Part model, mm, in its own coordinate system. Face numbers are marked on the shaded views. Give positions to 0.01 mm unless a question says otherwise; leave off trailing zeros. Write each loop counter-clockwise with the first axis right and the second up, starting at its lowest first coordinate (ties: lowest second). Pieces come first, ordered by that corner, then holes. Notation, with made-up numbers: (43, 70.5) - (76, 70.5) arc R35 ccw to (76, 103.5) - close; hole circle Ø7 at (89.5, 27.25). An arc over 180 degrees is marked (long way). Answer in a Markdown table with one row per item. Add a question column.
1. Band-saw the part on C-C on x = 13. Write the cut outline in (y, z), plus the area to 3 significant figures.
2. Band-saw the part on D-D on y = 15. Write the cut outline in (x, z), plus the area to 3 significant figures.
3. Pull direction X, two halves, no side cores. Call the marked faces 1, 2, 3 and 4: released by +X, released by -X, zero draft, split by the parting line, or undercut.
4. Drop flat-ended pins along their axis: pin 1 Ø8 at (x, y) = (4.5, 30.5) entering from +Z; pin 2 Ø6 at (x, y) = (14.5, 41) entering from +Z. Give the stop position or say it passes through.
5. Probe line 1 along X through (y, z) = (23.5, 11); line 2 along Z through (x, y) = (7.5, 15.5); line 3 along Y through (x, z) = (0.9, 36). List the from-to ranges inside material, lowest first.
6. Band-saw the part on A-A on z = 11.5. Write the cut outline in (x, y), plus the area to 3 significant figures.
7. Band-saw the part on B-B on y = 8. Write the cut outline in (x, z), plus the area to 3 significant figures.
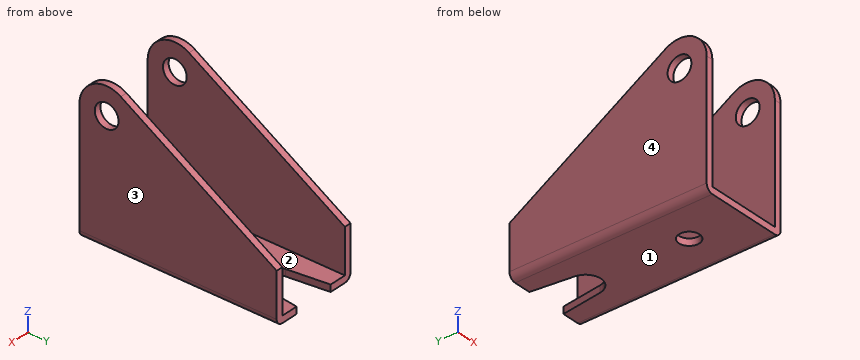
Autodesk Inventor part; units mm, degrees
ref_plane "YZ Plane" through (0, 0, 0) normal (1, 0, 0) x (0, 1, 0)
ref_plane "XZ Plane" through (0, 0, 0) normal (0, 1, 0) x (-1, 0, 0)
ref_plane "XY Plane" through (0, 0, 0) normal (0, 0, 1) x (1, 0, 0)
sketch "Sketch1" plane through (0, 0, 0) normal (0, 0, 1) x (1, 0, 0)
  line L0 (0, 0) -> (26, 0)
  line L1 (26, 0) -> (26, 58)
  line L2 (26, 58) -> (0, 58) construction
  line L3 (0, 58) -> (0, 0)
  circle A0 centre (13, 16) radius 3
  line L4 (0, 58) -> (7, 58)
  line L5 (19, 58) -> (26, 58)
  line L6 (17.464, 45.9318) -> (19, 58)
  line L7 (8.536, 45.9318) -> (7, 58)
  line L8 (13, 58) -> (13, 46.5) construction
  circle A1 centre (13, 46.5) radius 4.5 construction
  arc A2 (8.536, 45.9318) -> (17.464, 45.9318) centre (13, 46.5) ccw
  point P0 (13, 0)
  dimension "d0" = 26
  dimension "d1" = 58
  dimension "d2" = 6
  dimension "d3" = 16
  dimension "d19" = 12
  dimension "d20" = 9
  dimension "d21" = 11.5
extrude "Extrusion1" add sketch "Sketch1" along normal blind 2
sketch "Sketch2" plane through (26, 0, 0) normal (1, 0, 0) x (0, 0, -1)
  circle A0 centre (-36, 8) radius 3.5
  line L0 (0, 0) -> (0, 58)
  line L1 (0, 0) -> (-36, 0)
  circle A1 centre (-36, 8) radius 8 construction
  line L2 (0, 58) -> (-15, 58)
  line L3 (-15, 58) -> (-42.8382, 12.152)
  arc A2 (-42.8382, 12.152) -> (-36, 0) centre (-36, 8) ccw
  dimension "d13" = 16
  dimension "d8" = 7
  dimension "d10" = 8
  dimension "d11" = 36
  dimension "d14" = 15
extrude "Extrusion2" add sketch "Sketch2" against normal blind 2
sketch "Sketch3" plane through (0, 0, 0) normal (-1, 0, 0) x (0, 0, 1)
  line L0 (2, 0) -> (2, 58)
  line L1 (2, 0) -> (36, 0)
  arc A0 (36, 0) -> (42.8382, 12.152) centre (36, 8) ccw
  line L2 (42.8382, 12.152) -> (15, 58)
  line L3 (15, 58) -> (2, 58)
  circle A1 centre (36, 8) radius 3.5
  point P0 (0, 0)
extrude "Extrusion3" add sketch "Sketch3" against normal blind 2
fillet "Fillet1" radius 2 2 edges at (0, 29, 0) (26, 29, 0)
properties part number "Mount" material "Stainless Steel"
Values:
| question | item | result |
|---|---|---|
| 1 | outline | (0, 0) - (13, 0) - (13, 2) - (0, 2) - close; (19, 0) - (42, 0) - (42, 2) - (19, 2) - close |
| 1 | area | 72.0 mm² |
| 2 | outline | (0, 2) arc R2 ccw to (2, 0) - (10.17, 0) - (10.17, 2) - (2, 2) - (2, 41.11) - (0, 41.11) - close; (15.83, 0) - (24, 0) arc R2 ccw to (26, 2) - (26, 41.11) - (24, 41.11) - (24, 2) - (15.83, 2) - close |
| 2 | area | 195 mm² |
| 3 | face 1 | zero draft |
| 3 | face 2 | undercut |
| 3 | face 3 | released by +X |
| 3 | face 4 | released by -X |
| 4 | pin 1 | stops at z = 33.59 |
| 4 | pin 2 | stops at z = 2 |
| 5 | line 1 | x = 0 to 2, 24 to 26 |
| 5 | line 2 | z = 0 to 2 |
| 5 | line 3 | y = 0 to 4.5, 11.5 to 23.41 |
| 6 | outline | (0, 0) - (2, 0) - (2, 58) - (0, 58) - close; (24, 0) - (26, 0) - (26, 58) - (24, 58) - close |
| 6 | area | 232 mm² |
| 7 | outline | (0, 2) arc R2 ccw to (2, 0) - (24, 0) arc R2 ccw to (26, 2) - (26, 32.5) - (24, 32.5) - (24, 2) - (2, 2) - (2, 32.5) - (0, 32.5) - close; (0, 39.5) - (2, 39.5) - (2, 44) - (0, 44) - close; (24, 39.5) - (26, 39.5) - (26, 44) - (24, 44) - close |
| 7 | area | 190 mm² |
